Model file for the job. Use its own axes, mm. Face numbers are marked on the shaded views. A direction names the side the tool comes from. Round coordinates to 2 decimals unless told otherwise and drop trailing zeros. Order: outer loops, then holes, each group sorted by start corner. A loop starts at its lowest first (then second) coordinate and runs counter-clockwise, first axis right, second up. Notation, with made-up numbers: (83.25, -38.75) -> (113.25, -38.75) arc R17 cw to (113.25, -30.75) -> close; hole circle Ø4 at (7, 86.5). An arc over 180 degrees is marked (long way). Answer as CSV lines item,"result".
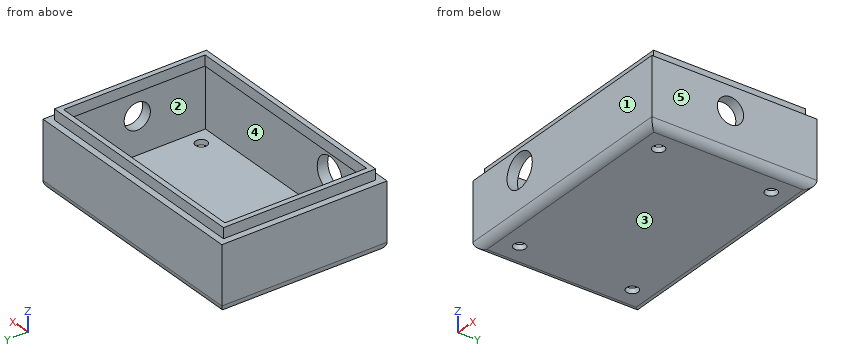
```python
from build123d import *

# Parameters (mm, degrees)
SKETCH3_W           = 92
SKETCH3_H           = 63
SKETCH3_R           = 2.25
BOSS_EXTRUDE3_DEPTH = 25
SKETCH4_W           = 84
SKETCH4_H           = 55
CUT_EXTRUDE1_DEPTH  = 23
FILLET1_R           = 3
SKETCH5_W           = 87
SKETCH5_H           = 58
BOSS_EXTRUDE4_DEPTH = 4
SKETCH7_W           = 83
SKETCH7_H           = 54
CUT_EXTRUDE4_DEPTH  = 27
SKETCH9_R           = 6.5
CUT_EXTRUDE6_DEPTH  = 27
SKETCH11_R          = 5
CUT_EXTRUDE7_DEPTH  = 27


with BuildPart() as part:
    # Sketch3 → Boss-Extrude3 (new body)
    with BuildSketch(Plane.XY):
        with Locations((46, 31.5)):
            Rectangle(SKETCH3_W, SKETCH3_H)
        with Locations((82, 53)):
            Circle(SKETCH3_R, mode=Mode.SUBTRACT)
        with Locations((82, 10)):
            Circle(SKETCH3_R, mode=Mode.SUBTRACT)
        with Locations((10.5, 10)):
            Circle(SKETCH3_R, mode=Mode.SUBTRACT)
        with Locations((10.5, 53)):
            Circle(SKETCH3_R, mode=Mode.SUBTRACT)
    extrude(amount=BOSS_EXTRUDE3_DEPTH)

    # Sketch4 → Cut-Extrude1 (cut)
    with BuildSketch(Plane.XY.offset(25)):
        with Locations((46, 31.5)):
            Rectangle(SKETCH4_W, SKETCH4_H)
    extrude(amount=-CUT_EXTRUDE1_DEPTH, mode=Mode.SUBTRACT)

    # Fillet1
    fillet1_edges = [part.edges().sort_by_distance(p)[0] for p in [
        (46, 63, 0),
        (92, 31.5, 0),
        (46, 0, 0),
        (0, 31.5, 0),
    ]]
    fillet(fillet1_edges, radius=FILLET1_R)

    # Sketch5 → Boss-Extrude4 (add)
    with BuildSketch(Plane.XY.offset(25)):
        with Locations((46, 31.5)):
            Rectangle(SKETCH5_W, SKETCH5_H)
    extrude(amount=BOSS_EXTRUDE4_DEPTH)

    # Sketch7 → Cut-Extrude4 (cut)
    with BuildSketch(Plane.XY.offset(29)):
        with Locations((46, 31.5)):
            Rectangle(SKETCH7_W, SKETCH7_H)
    extrude(amount=-CUT_EXTRUDE4_DEPTH, mode=Mode.SUBTRACT)

    # Sketch9 → Cut-Extrude6 (cut)
    with BuildSketch(Plane.XZ):
        with Locations(Location((24, 17, 0), (0, 0, 270))):
            Circle(SKETCH9_R)
    extrude(amount=-CUT_EXTRUDE6_DEPTH, mode=Mode.SUBTRACT)

    # Sketch11 → Cut-Extrude7 (cut)
    with BuildSketch(Plane(origin=(92, 0, 0), x_dir=(0, 0, -1), z_dir=(1, 0, 0))):
        with Locations((-16, 30)):
            Circle(SKETCH11_R)
    extrude(amount=-CUT_EXTRUDE7_DEPTH, mode=Mode.SUBTRACT)


solid = part.part
```
Q1. Saw through at D-D (y = 53). Write the cut outline in (x, z).
Checks:
outline,"(0, 3) arc R3 ccw to (3, 0) -> (8.25, 0) -> (8.25, 2) -> (4, 2) -> (4, 25) -> (4.5, 25) -> (4.5, 29) -> (2.5, 29) -> (2.5, 25) -> (0, 25) -> close; (12.75, 0) -> (79.75, 0) -> (79.75, 2) -> (12.75, 2) -> close; (84.25, 0) -> (89, 0) arc R3 ccw to (92, 3) -> (92, 25) -> (89.5, 25) -> (89.5, 29) -> (87.5, 29) -> (87.5, 25) -> (88, 25) -> (88, 2) -> (84.25, 2) -> close"
Q2. Mould opens along X. For the marked faces 3, 4 and 5 say: +X half, -X half, draft (parallel to the pull), parting line (faces both ways), or undercut.
Checks:
face 3,"draft"
face 4,"undercut"
face 5,"+X half"
Q3. Flat gauge pins, fed straight in: pin 1 (1.2 mm diameter, centred on y = 18, z = 26.5, fed in from -X); pin 2 (3 mm diameter, centred on y = 45, z = 28, fed in from +X); pin 3 (2.5 mm diameter, centred on x = 82, y = 53, fed in from -Z); pin 4 (10.5 mm diameter, centred on x = 24, z = 17, fed in from -Y). Where does each tip first touch, or does it go through?
Checks:
pin 1,"x = 2.5"
pin 2,"x = 89.5"
pin 3,"through"
pin 4,"y = 59"
Q4. Saw through at A-A (y = 30). Write the cut outline in (x, z), plus the area to 3 significant figures.
Checks:
outline,"(0, 3) arc R3 ccw to (3, 0) -> (89, 0) arc R3 ccw to (92, 3) -> (92, 11) -> (88, 11) -> (88, 2) -> (4, 2) -> (4, 25) -> (4.5, 25) -> (4.5, 29) -> (2.5, 29) -> (2.5, 25) -> (0, 25) -> close; (87.5, 25) -> (88, 25) -> (88, 21) -> (92, 21) -> (92, 25) -> (89.5, 25) -> (89.5, 29) -> (87.5, 29) -> close"
area,"340 mm²"
Q5. Tool access for the marked faces 1 and 2: list every direction of +Z, -Z, +X, -X, +Y, -Y with a clear straight run to the whole face (end or side of a thin tool).
Checks:
face 1,"+Z, -Z, +X, -X, -Y"
face 2,"none"
Q6. Saw through at B-B (x = 10.5). Write the cut outline in (y, z), plus the area to 3 significant figures.
Checks:
outline,"(0, 3) arc R3 ccw to (3, 0) -> (7.75, 0) -> (7.75, 2) -> (4, 2) -> (4, 25) -> (4.5, 25) -> (4.5, 29) -> (2.5, 29) -> (2.5, 25) -> (0, 25) -> close; (12.25, 0) -> (50.75, 0) -> (50.75, 2) -> (12.25, 2) -> close; (55.25, 0) -> (60, 0) arc R3 ccw to (63, 3) -> (63, 25) -> (60.5, 25) -> (60.5, 29) -> (58.5, 29) -> (58.5, 25) -> (59, 25) -> (59, 2) -> (55.25, 2) -> close"
area,"304 mm²"
Q7. Wall check: L1, parallel to Y at x = 8.5, z = 9.5; L2, parallel to X at y = 34, z = 5.75; L3, parallel to Y at x = 82, z = 1.25. Give the ranges that are in metal, low to high. Write a range as [from, to].
Checks:
L1,"[0, 4], [59, 63]"
L2,"[0, 4], [88, 92]"
L3,"[0.56, 7.75], [12.25, 50.75], [55.25, 62.44]"
Q8. Saw through at C-C (x = 24). Write the cut outline in (y, z).
Checks:
outline,"(0, 3) arc R3 ccw to (3, 0) -> (60, 0) arc R3 ccw to (63, 3) -> (63, 25) -> (60.5, 25) -> (60.5, 29) -> (58.5, 29) -> (58.5, 25) -> (59, 25) -> (59, 2) -> (4, 2) -> (4, 10.5) -> (0, 10.5) -> close; (0, 23.5) -> (4, 23.5) -> (4, 25) -> (4.5, 25) -> (4.5, 29) -> (2.5, 29) -> (2.5, 25) -> (0, 25) -> close"
